from build123d import *

# Parameters (mm, degrees)
LID_PLATE_START               = 88
SKETCH1_W                     = 166
SKETCH1_H                     = 106
LID_PLATE_DEPTH               = 3
TFT_WINDOW_DEPTH              = 135.085793431
TFT_WINDOW_DEPTH_BACK         = 135.085793431
SKETCH2_W                     = 35.4
SKETCH2_H                     = 28.4
LID_SCREW_HOLES_M3_DEPTH      = 135.085793431
LID_SCREW_HOLES_M3_DEPTH_BACK = 135.085793431
SKETCH3_R                     = 1.7
TFT_RAILS_START               = 88
SKETCH4_W                     = 48
SKETCH4_H                     = 2
TFT_RAILS_DEPTH               = 5.8
TFT_RAIL_LIPS_START           = 83.2
SKETCH5_W                     = 48
SKETCH5_H                     = 1.2
TFT_RAIL_LIPS_DEPTH           = 1


with BuildPart() as part:
    # Sketch1 → Lid_Plate (new body)
    with BuildSketch(Plane(origin=(0, 0, 0), x_dir=(1, 0, 0), z_dir=(0, 1, 0)).offset(LID_PLATE_START)):
        Rectangle(SKETCH1_W, SKETCH1_H)
    extrude(amount=LID_PLATE_DEPTH)

    # Sketch2 → TFT_Window (cut, two sides: drawn at the far end of the back side and taken through both)
    with BuildSketch(Plane(origin=(0, 0, 0), x_dir=(1, 0, 0), z_dir=(0, 1, 0)).offset(-TFT_WINDOW_DEPTH_BACK)):
        with Locations((20, -8)):
            Rectangle(SKETCH2_W, SKETCH2_H)
    extrude(amount=TFT_WINDOW_DEPTH + TFT_WINDOW_DEPTH_BACK, mode=Mode.SUBTRACT)

    # Sketch3 → Lid_Screw_Holes_M3 (cut, two sides: drawn at the far end of the back side and taken through both)
    with BuildSketch(Plane(origin=(0, 0, 0), x_dir=(1, 0, 0), z_dir=(0, 1, 0)).offset(-LID_SCREW_HOLES_M3_DEPTH_BACK)):
        with Locations(Location((-76, 46, 0), (0, 0, 270))):
            Circle(SKETCH3_R)
        with Locations(Location((-76, -46, 0), (0, 0, 270))):
            Circle(SKETCH3_R)
        with Locations(Location((76, 46, 0), (0, 0, 270))):
            Circle(SKETCH3_R)
        with Locations(Location((76, -46, 0), (0, 0, 270))):
            Circle(SKETCH3_R)
    extrude(amount=LID_SCREW_HOLES_M3_DEPTH + LID_SCREW_HOLES_M3_DEPTH_BACK, mode=Mode.SUBTRACT)

    # Sketch4 → TFT_Rails (add)
    with BuildSketch(Plane(origin=(0, 0, 0), x_dir=(1, 0, 0), z_dir=(0, 1, 0)).offset(TFT_RAILS_START)):
        with Locations((20, 10.8)):
            Rectangle(SKETCH4_W, SKETCH4_H)
        with Locations((20, -26.8)):
            Rectangle(SKETCH4_W, SKETCH4_H)
    extrude(amount=-TFT_RAILS_DEPTH)

    # Sketch5 → TFT_Rail_Lips (add)
    with BuildSketch(Plane(origin=(0, 0, 0), x_dir=(1, 0, 0), z_dir=(0, 1, 0)).offset(TFT_RAIL_LIPS_START)):
        with Locations((20, 9.2)):
            Rectangle(SKETCH5_W, SKETCH5_H)
        with Locations((20, -25.2)):
            Rectangle(SKETCH5_W, SKETCH5_H)
    extrude(amount=-TFT_RAIL_LIPS_DEPTH)


solid = part.part
For this review, take the finished solid that the model builds, in its own axes (mm). A direction names the side the tool comes from. Round coordinates to 2 decimals unless told otherwise and drop trailing zeros. Write each loop counter-clockwise with the first axis right and the second up, starting at its lowest first coordinate (ties: lowest second). Pieces come first, ordered by that corner, then holes. Notation, with made-up numbers: (-21, 13.5) -> (-5, 13.5) arc R14 cw to (-5, 38.5) -> close; hole circle Ø7 at (72.25, -36). An arc over 180 degrees is marked (long way). Put each result on its own line as item: value.
Q1. The part is to be moulded in two halves that separate along Z. For faces 4 (the flat face through (20, 85, -11.8)), 5 (the flat face through (44, 85, -11)), 6 (the flat face through (20, 89, -6.2)), say which applies: released by +Z, released by -Z, zero draft, split by the parting line, or undercut.
Determined:
face 4: released by -Z
face 5: zero draft
face 6: undercut
Q2. Clearance check with flat-ended pins moving along their axes: pin 1 Ø0.8 at (x, y) = (21.5, 82.5) entering from +Z; pin 2 Ø0.5 at (x, y) = (31, 83) entering from -Z; pin 3 Ø5.5 at (x, z) = (-76, -46) entering from -Y. State where each tip first meets the part, or that it passes through.
Determined:
pin 1: stops at z = 27.8
pin 2: stops at z = -11.8
pin 3: stops at y = 88
Q3. Consider section A-A on y = 85.5. State the section outline as (x, z) points.
Determined:
outline: (-4, -11.8) -> (44, -11.8) -> (44, -9.8) -> (-4, -9.8) -> close; (-4, 25.8) -> (44, 25.8) -> (44, 27.8) -> (-4, 27.8) -> close
Q4. Machinability: for faces 1 (the flat face through (20, 86, -9.8)), 2 (the flat face through (20, 85, 27.8)), 3 (the flat face through (2.3, 89, 8)), which of the approach directions +Z, -Z, +X, -X, +Y, -Y give a long, thin tool a straight path to every point of the face, cutting with its end or side? Answer none if there is none.
Determined:
face 1: +X, -X
face 2: +Z, +X, -X, -Y
face 3: +Y, -Y
Q5. Consider section D-D on x = -76. State the section outline as (y, z) points, and give its area (3 significant figures).
Determined:
outline: (88, -53) -> (91, -53) -> (91, -47.7) -> (88, -47.7) -> close; (88, -44.3) -> (91, -44.3) -> (91, 44.3) -> (88, 44.3) -> close; (88, 47.7) -> (91, 47.7) -> (91, 53) -> (88, 53) -> close
area: 298 mm^2
Q6. Consider section C-C on x = 11. State the section outline as (y, z) points, and give its area (3 significant figures).
Determined:
outline: (82.2, -11.8) -> (88, -11.8) -> (88, -53) -> (91, -53) -> (91, -6.2) -> (88, -6.2) -> (88, -9.8) -> (83.2, -9.8) -> (83.2, -8.6) -> (82.2, -8.6) -> close; (82.2, 24.6) -> (83.2, 24.6) -> (83.2, 25.8) -> (88, 25.8) -> (88, 22.2) -> (91, 22.2) -> (91, 53) -> (88, 53) -> (88, 27.8) -> (82.2, 27.8) -> close
area: 258 mm^2
Q7. To check wall thickness, follow L1, parallel to Z at x = -76, y = 89; L2, parallel to X at y = 90.25, z = 46; L3, parallel to Y at x = 31.5, z = -9.5. State the ranges of each line that lie inside material, in increasing order. Write a range as [from, to].
Determined:
L1: z = [-53, -47.7], [-44.3, 44.3], [47.7, 53]
L2: x = [-83, -77.7], [-74.3, 74.3], [77.7, 83]
L3: y = [82.2, 83.2], [88, 91]
Q8. Consider section B-B on z = -46. State the section outline as (x, y) points, and give its area (3 significant figures).
Determined:
outline: (-83, 88) -> (-77.7, 88) -> (-77.7, 91) -> (-83, 91) -> close; (-74.3, 88) -> (74.3, 88) -> (74.3, 91) -> (-74.3, 91) -> close; (77.7, 88) -> (83, 88) -> (83, 91) -> (77.7, 91) -> close
area: 478 mm^2
